Could you check a few things on this model? Use its own coordinates, in mm. Face numbers are marked on the shaded views. A direction names the side the tool comes from. Give positions to 0.01 mm unless a question says otherwise; leave off trailing zeros. Order: outer loops, then holes, each group sorted by start corner. A loop starts at its lowest first (then second) coordinate and runs counter-clockwise, first axis right, second up. Notation, with made-up numbers: (-11, -6) -> (7, -6) arc R25 cw to (7, 12) -> close; hole circle Ø8 at (-38.75, 56). An arc over 180 degrees is marked (long way). One line per item, written item: value.
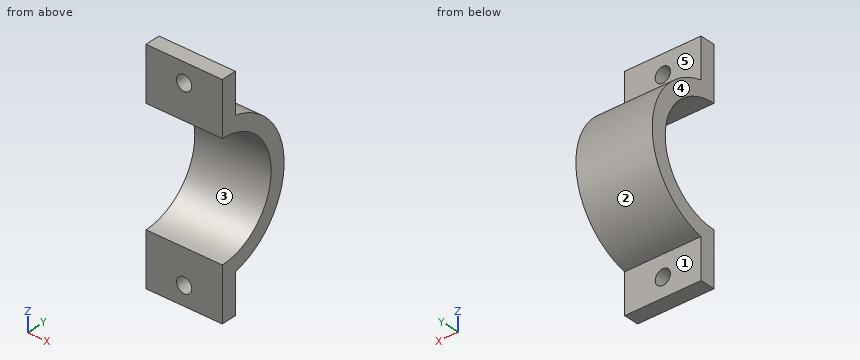
```python
from build123d import *

# Parameters (mm, degrees)
BOSS_EXTRUDE1_DEPTH = 10
SKETCH2_R           = 1
CUT_EXTRUDE1_DEPTH  = 2
SKETCH3_R           = 1
CUT_EXTRUDE5_DEPTH  = 2


with BuildPart() as part:
    # Sketch1 → Boss-Extrude1 (new body)
    with BuildSketch(Plane(origin=(0, 0, 0), x_dir=(0, 0, -1), z_dir=(1, 0, 0))):
        with BuildLine():
            Line((7.5, 0), (14.5, 0))
            Line((14.5, 0), (14.5, 2))
            Line((14.5, 2), (9.287087811, 2))
            ThreePointArc((9.287087811, 2), (0, 9.5), (-9.287087811, 2))
            Line((-9.287087811, 2), (-14.5, 2))
            Line((-14.5, 2), (-14.5, 0))
            Line((-14.5, 0), (-7.5, 0))
            ThreePointArc((-7.5, 0), (0, 7.5), (7.5, 0))
        make_face()
    extrude(amount=BOSS_EXTRUDE1_DEPTH)

    # Sketch2 → Cut-Extrude1 (cut)
    with BuildSketch(Plane(origin=(0, 2, 0), x_dir=(1, 0, 0), z_dir=(0, 1, 0))):
        with Locations(Location((5, 12, 0), (0, 0, 270))):
            Circle(SKETCH2_R)
    extrude(amount=-CUT_EXTRUDE1_DEPTH, mode=Mode.SUBTRACT)

    # Sketch3 → Cut-Extrude5 (cut)
    with BuildSketch(Plane(origin=(0, 0, 0), x_dir=(1, 0, 0), z_dir=(0, 1, 0))):
        with Locations(Location((5, -12, 0), (0, 0, 270))):
            Circle(SKETCH3_R)
    extrude(amount=CUT_EXTRUDE5_DEPTH, mode=Mode.SUBTRACT)


solid = part.part
```
1) Suppose I cut it at A-A, the plane z = -12. Write out the boundary of the cut face in (x, y), then the cut area to 3 significant figures.
Answer below:
outline: (0, 0) -> (4, 0) -> (4, 2) -> (0, 2) -> close; (6, 0) -> (10, 0) -> (10, 2) -> (6, 2) -> close
area: 16.0 mm2
2) For the marked faces 4 and 5, which set-ups out of +Z, -Z, +X, -X, +Y, -Y let a thin tool reach every point of the face, with its end or its side?
Answer below:
face 4: +Z, -Z, -X, +Y, -Y
face 5: +Z, +X, -X, +Y
3) Suppose I cut it at C-C, the plane y = 4.5. Write out the boundary of the cut face in (x, z), then the cut area to 3 significant figures.
Answer below:
outline: (0, -8.37) -> (10, -8.37) -> (10, -6) -> (0, -6) -> close; (0, 6) -> (10, 6) -> (10, 8.37) -> (0, 8.37) -> close
area: 47.3 mm2
4) Suppose I cut it at B-B, the plane x = 5. Write out the boundary of the cut face in (y, z).
Answer below:
outline: (0, -14.5) -> (2, -14.5) -> (2, -13) -> (0, -13) -> close; (0, -11) -> (2, -11) -> (2, -9.29) arc R9.5 ccw to (2, 9.29) -> (2, 11) -> (0, 11) -> (0, 7.5) arc R7.5 cw to (0, -7.5) -> close; (0, 13) -> (2, 13) -> (2, 14.5) -> (0, 14.5) -> close
5) For P1, Ø1, axis at x = 7.5, z = -1.5, coming from the -Y side; P2, Ø2, axis at x = 8, z = 10.5, coming from the +Y side; P3, Ø4, axis at x = 4, z = 7.5, coming from the +Y side; P4, Ø3, axis at x = 5, z = 12, coming from the -Y side, each with a flat end and sliding along its axis, tell me the tip position at first contact or that it passes through.
Answer below:
P1: stops at y = 7.23
P2: stops at y = 2
P3: stops at y = 7.75
P4: stops at y = 0
6) If I drill on line 1 along X through (y, z) = (1.5, 12); line 2 along Y through (x, z) = (2.5, 12.75); line 3 along Z through (x, y) = (9, 1.75), over which ranges is the centre line in solid material (lowest first)?
Answer below:
line 1: x = 0 to 4, 6 to 10
line 2: y = 0 to 2
line 3: z = -14.5 to -7.29, 7.29 to 14.5
7) We'd pull the mould along Z, two halves only. Please class the marked faces 1, 2 and 3: +Z half, -Z half, draft (parallel to the pull), parting line (faces both ways), or undercut.
Answer below:
face 1: draft
face 2: parting line
face 3: undercut
8) Suppose I cut it at D-D, the plane x = 7.25. Write out the boundary of the cut face in (y, z).
Answer below:
outline: (0, -14.5) -> (2, -14.5) -> (2, -9.29) arc R9.5 ccw to (2, 9.29) -> (2, 14.5) -> (0, 14.5) -> (0, 7.5) arc R7.5 cw to (0, -7.5) -> close
